Autodesk Inventor part; units mm, degrees
ref_plane "Work Plane6" through (21, 0, 40) normal (0, 0, -1) x (-1, 0, 0)
ref_plane "YZ Plane" through (0, 0, 0) normal (1, 0, 0) x (0, 1, 0)
ref_plane "XZ Plane" through (0, 0, 0) normal (0, 1, 0) x (-1, 0, 0)
sketch "Sketch1" plane through (0, 0, 0) normal (0, 0, 1) x (1, 0, 0)
  point P0 (0, 0)
sketch "Sketch2" plane through (0, 0, 0) normal (0, 0, 1) x (1, 0, 0)
  line L0 (0, 0) -> (-21, 0)
  line L1 (0, 0) -> (21, 0)
  line L2 (21, -70) -> (-21, -70)
  line L3 (-21, -70) -> (-35, -70)
  line L4 (-35, -70) -> (-21, 0)
  line L5 (21, -70) -> (35, -70)
  line L6 (35, -70) -> (21, 0)
  line L7 (-35, -70) -> (-36.4709, -69.7058)
  line L8 (-22.4709, 0.2942) -> (-36.4709, -69.7058)
  line L9 (-22.4709, 0.2942) -> (-22.2297, 1.5)
  line L10 (35, -70) -> (36.4709, -69.7058)
  line L11 (22.4709, 0.2942) -> (36.4709, -69.7058)
  line L12 (-22.2297, 1.5) -> (22.2297, 1.5)
  line L13 (22.2297, 1.5) -> (22.4709, 0.2942)
  dimension "d3" = 21
  dimension "d4" = 21
  dimension "d5" = 70
  dimension "d6" = 14
  dimension "d7" = 14
  dimension "d24" = 1.5
  dimension "d25" = 1.5
  dimension "d26" = 1.5
extrude "Extrusion1" add sketch "Sketch2" along normal blind 45 contours L0 L4 L7 L8 L9 L12 L13 L11 L10 L6 L1
sketch "Sketch3" plane through (-21, 0, 0) normal (0, -1, 0) x (1, 0, 0)
  point P0 (21, 0)
sketch "Sketch5" plane through (-21, 0, 0) normal (0, -1, 0) x (1, 0, 0)
  line L0 (0, 45) -> (42, 45)
  line L1 (19.4909, 45) -> (14.4909, 45)
  line L2 (24.3761, 45) -> (24.3761, 40)
  line L3 (24.3761, 40) -> (42, 40)
  line L4 (42, 40) -> (0, 40)
  point P0 (21, 0)
  dimension "d16" = 5
  dimension "d17" = 5
sketch "Sketch6" plane through (-21, 0, 0) normal (0, -1, 0) x (1, 0, 0)
  point P0 (21, 0)
ref_plane "Work Plane6" through (21, 0, 40) normal (0, 0, -1) x (-1, 0, 0)
sketch "Sketch7" plane through (21, 0, 40) normal (0, 0, -1) x (-1, 0, 0)
  line L0 (42, 0) -> (0, 0)
  line L1 (0, 0) -> (42, 0)
  line L2 (42, -25) -> (47, -25)
  line L3 (56, -70) -> (42, 0)
  line L4 (42, -25) -> (-5, -25)
  line L5 (0, 0) -> (-14, -70)
  line L6 (0, 0) -> (-5, -25)
  line L7 (47, -25) -> (42, 0)
  line L8 (44.0495, 2.5) -> (58.4515, -69.5097)
  line L9 (47, -25) -> (42, -25)
  point P0 (21, 0)
  dimension "d19" = 25
extrude "Extrusion3" add sketch "Sketch7" against normal blind 1.5
sketch "Sketch8" plane through (0, 0, 0) normal (0, 0, -1) x (-1, 0, 0)
  point P0 (0, 0)
sketch "Sketch9" plane through (0, 0, 0) normal (0, 0, -1) x (-1, 0, 0)
  line L0 (-36.4709, -69.7058) -> (-22.2297, 1.5)
  line L1 (36.4709, -69.7058) -> (-36.4709, -69.7058)
  line L2 (-36.4709, -69.7058) -> (-22.2297, 1.5)
  line L3 (-22.2297, 1.5) -> (22.2297, 1.5)
  line L4 (22.2297, 1.5) -> (36.4709, -69.7058)
  line L5 (22.2297, 1.5) -> (36.4709, -69.7058)
  line L6 (22.2297, 1.5) -> (36.4709, -69.7058)
  line L7 (36.4709, -69.7058) -> (36.4709, -69.7058)
  point P0 (0, 0)
extrude "Extrusion4" add sketch "Sketch9" along normal blind 1.5
properties part number "Modulo"
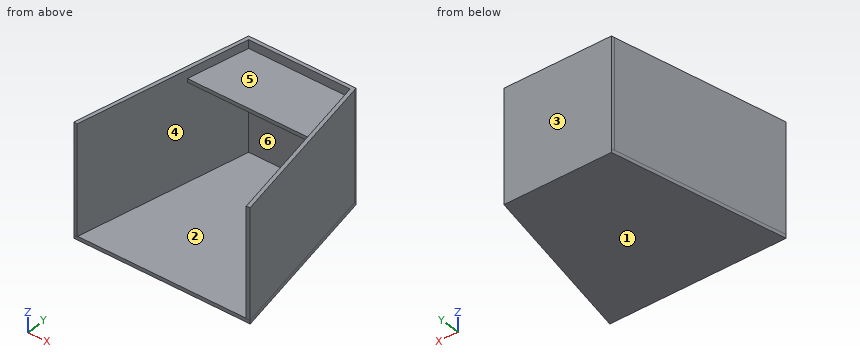
The listing builds one solid part. Answer for the finished solid, in the listing's coordinates (mm). Face numbers are marked on the shaded views. A direction names the side the tool comes from. Round coordinates to 2 decimals unless told otherwise and drop trailing zeros. Loops run counter-clockwise (first coordinate to the right, second up) from the corner with the lowest first, then second, coordinate; pieces in that order, holes last. Notation, with made-up numbers: (54, -18.5) -> (102, -18.5) arc R21 cw to (102, 20.5) -> close; hole circle Ø11 at (-26, -26). An arc over 180 degrees is marked (long way). Use one line per item in the form item = value.
1. Flat-ended cylindrical pins translate along their axes: pin 1 Ø12 at (y, z) = (-61.5, 13) entering from -X; pin 2 Ø1.6 at (x, z) = (8.5, 40.5) entering from -Y; pin 3 Ø0.8 at (x, z) = (8, -0.5) entering from -Y. Find the tip coordinate at first contact, or state that the pin passes through.
Answer key:
pin_1 = -36.03
pin_2 = -25
pin_3 = -69.71
2. The part is cut by section B-B on x = 13. Determine the outline of the cut face in (y, z), and give its area (3 significant figures).
Answer key:
outline = (-69.71, -1.5) -> (1.5, -1.5) -> (1.5, 45) -> (0, 45) -> (0, 41.5) -> (-25, 41.5) -> (-25, 40) -> (0, 40) -> (0, 0) -> (-69.71, 0) -> close
area = 212 mm²
3. The part is cut by section A-A on z = 27.5. Determine the outline of the cut face in (x, y).
Answer key:
outline = (-36.47, -69.71) -> (-35, -70) -> (-21, 0) -> (21, 0) -> (35, -70) -> (36.47, -69.71) -> (22.47, 0.29) -> (22.23, 1.5) -> (-22.23, 1.5) -> (-22.47, 0.29) -> close
4. For a pull along Z with two mould halves and no side action, classify the marked faces 3, 4, 5 and 6 as released by +Z, released by -Z, zero draft, split by the parting line, or undercut.
Answer key:
face_3 = zero draft
face_4 = undercut
face_5 = released by +Z
face_6 = undercut
5. Find the intervals of material crossed by probe 1 along Z at (x, y) = (-13, -1.5); probe 2 along Z at (x, y) = (23, -27.5); probe 3 along Y at (x, z) = (-5.5, 10.5), in increasing order. Write a range as [from, to].
Answer key:
probe_1 = [-1.5, 0], [40, 41.5]
probe_2 = [-1.5, 0]
probe_3 = [0, 1.5]
6. A tool of negligible diameter and unlimited length cuts with its end or side. For the marked faces 1 and 2, from which of +Z, -Z, +X, -X, +Y, -Y can it reach the whole face along a straight path? Write none if from no direction.
Answer key:
face_1 = -Z, +X, -X, +Y, -Y
face_2 = -Y
